The listing builds one solid part. Answer for the finished solid, in the listing's coordinates (mm). Face numbers are marked on the shaded views. Round coordinates to 2 decimals unless told otherwise and drop trailing zeros. Loops run counter-clockwise (first coordinate to the right, second up) from the corner with the lowest first, then second, coordinate; pieces in that order, holes last. Notation, with made-up numbers: M -21.75,-38 L 19.25,-38 A24 cw 19.25,-23 Z; hole C 25.5,11 d11. An arc over 180 degrees is marked long. Put each result on its own line as item: value. Start each with the question number.
(1) Straight lines are drawn through the part: line 1 (X direction, y = 5, z = 18); line 2 (X direction, y = 13.25, z = -47); line 3 (X direction, y = 18.75, z = -24.5). For each, find the intervals that lie inside material, in ascending order.
(2) Determine the mould class of the marked faces 1 and 2 for opening direction X: released by +X, released by -X, zero draft, split by the parting line, or undercut.
(3) Section B-B, the plane x = 0 is taken. Determine the outline of the cut face in (y, z).
(4) Flat-ended cylindrical pins translate along their axes: P1, Ø1, axis at x = 36.5, y = 6.5, coming from the +Z side; P2, Ø1, axis at x = -95.5, z = -94.5, coming from the +Y side; P3, Ø5, axis at y = 13.5, z = 75, coming from the +X side. Find the tip coordinate at first contact, or state that the pin passes through.
(5) Section A-A, the plane y = 18.25 is taken. Determine the outline of the cut face in (x, z).
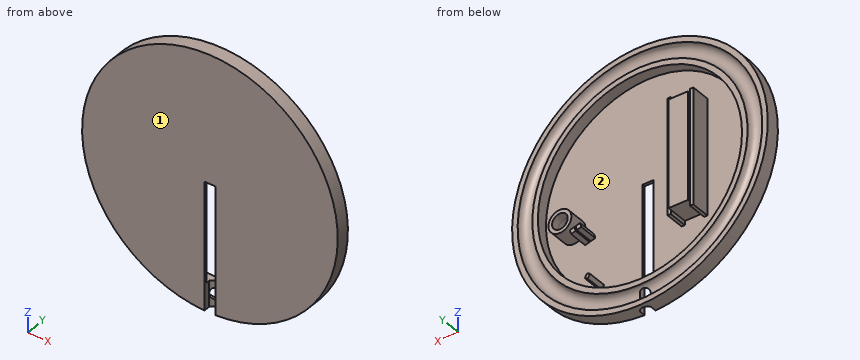
```python
from build123d import *

# Parameters (mm, degrees)
SKETCH1_W                = 139
SKETCH1_H                = 15
SKETCH4_W                = 21
SKETCH4_H                = 117
BOSS_EXTRUDE1_DEPTH      = 12
SKETCH5_R                = 12.5
SKETCH5_R_2              = 8.5
BOSS_EXTRUDE2_DEPTH      = 8.8
BOSS_EXTRUDE3_DEPTH      = 8.8
SKETCH11_W               = 28
SKETCH11_H               = 126
SKETCH11_W_2             = 21
SKETCH11_H_2             = 117
BOSS_EXTRUDE5_DEPTH      = 8.8
CUT_EXTRUDE1_START       = -12
SKETCH13_R               = 111
SKETCH13_R_2             = 12.5
SKETCH13_W               = 28
SKETCH13_H               = 126
SKETCH13_R_3             = 8.5
CUT_EXTRUDE1_DEPTH       = 12
BOSS_EXTRUDE6_DEPTH      = 8.8
BOSS_EXTRUDE6_DEPTH_BACK = 12
SKETCH14_W               = 21
SKETCH14_H               = 4.5
CUT_EXTRUDE2_DEPTH       = 20.8
CUT_EXTRUDE3_START       = -139
CUT_EXTRUDE3_DEPTH       = 139


# Read off the part's stored shape, not the designer's step: Cut-Extrude3
with BuildPart() as part:
    # Sketch1 → Revolve1 (revolve)
    with BuildSketch(Plane.XY, mode=Mode.PRIVATE) as revolve1_sk:
        with Locations((69.5, 7.5)):
            Rectangle(SKETCH1_W, SKETCH1_H)
    revolve(revolve1_sk.sketch.rotate(Axis((0, 4.511025306, 0), (0, 1, 0)), 90), axis=Axis((0, 4.511025306, 0), (0, 1, 0)))

    # Sketch4 → Boss-Extrude1 (add)
    with BuildSketch(Plane(origin=(0, 15, 0), x_dir=(1, 0, 0), z_dir=(0, 1, 0))):
        with Locations((-50.5, 0)):
            Rectangle(SKETCH4_W, SKETCH4_H)
    extrude(amount=BOSS_EXTRUDE1_DEPTH)

    # Sketch5 → Boss-Extrude2 (add)
    with BuildSketch(Plane(origin=(0, 15, 0), x_dir=(1, 0, 0), z_dir=(0, 1, 0))):
        with Locations(Location((80.590940898, 19.851958221, 0), (0, 0, 270))):
            Circle(SKETCH5_R)
        with Locations(Location((80.590940898, 19.851958221, 0), (0, 0, 270))):
            Circle(SKETCH5_R_2, mode=Mode.SUBTRACT)
    extrude(amount=BOSS_EXTRUDE2_DEPTH)

    # Sketch9 → Boss-Extrude3 (add)
    with BuildSketch(Plane(origin=(0, 15, 0), x_dir=(1, 0, 0), z_dir=(0, 1, 0))):
        with BuildLine():
            Line((47.886099404, 90.060654472), (50.233457218, 94.475392436))
            ThreePointArc((50.233457218, 94.475392436), (51.874629366, 93.584308664), (53.5, 92.664718205))
            Line((53.5, 92.664718205), (51, 88.334591186))
            ThreePointArc((51, 88.334591186), (49.450581265, 89.211210128), (47.886099404, 90.060654472))
        make_face()
    extrude(amount=BOSS_EXTRUDE3_DEPTH)

    # Sketch11 → Boss-Extrude5 (add)
    with BuildSketch(Plane(origin=(0, 15, 0), x_dir=(1, 0, 0), z_dir=(0, 1, 0))):
        with Locations((-50.5, 0)):
            Rectangle(SKETCH11_W, SKETCH11_H)
        with Locations((-50.5, 0)):
            Rectangle(SKETCH11_W_2, SKETCH11_H_2, mode=Mode.SUBTRACT)
    extrude(amount=BOSS_EXTRUDE5_DEPTH)

    # Sketch13 → Cut-Extrude1 (cut)
    # profile 1 of 2: a face of its own
    with BuildSketch(Plane(origin=(0, 15, 0), x_dir=(1, 0, 0), z_dir=(0, 1, 0)).offset(CUT_EXTRUDE1_START)):
        with Locations(Location((0, 0, 0), (0, 0, 270))):
            Circle(SKETCH13_R)
        with Locations(Location((80.590940898, 19.851958221, 0), (0, 0, 90))):
            Circle(SKETCH13_R_2, mode=Mode.SUBTRACT)
        with BuildLine():
            ThreePointArc((50.233457218, 94.475392436), (51.874629366, 93.584308664), (53.5, 92.664718205))
            Line((53.5, 92.664718205), (51, 88.334591186))
            ThreePointArc((51, 88.334591186), (49.450581265, 89.211210128), (47.886099404, 90.060654472))
            Line((47.886099404, 90.060654472), (50.233457218, 94.475392436))
        make_face(mode=Mode.SUBTRACT)
        with Locations((-50.5, 0)):
            Rectangle(SKETCH13_W, SKETCH13_H, mode=Mode.SUBTRACT)
    # profile 2 of 2: a face of its own
    with BuildSketch(Plane(origin=(0, 15, 0), x_dir=(1, 0, 0), z_dir=(0, 1, 0)).offset(CUT_EXTRUDE1_START)):
        with Locations(Location((80.590940898, 19.851958221, 0), (0, 0, 90))):
            Circle(SKETCH13_R_3)
    extrude(amount=CUT_EXTRUDE1_DEPTH, mode=Mode.SUBTRACT)

    # Sketch12 → Boss-Extrude6 (add, two sides: drawn at the far end of the back side and taken through both)
    with BuildSketch(Plane(origin=(0, 15, 0), x_dir=(1, 0, 0), z_dir=(0, 1, 0)).offset(-BOSS_EXTRUDE6_DEPTH_BACK)):
        Polygon((64.928294207, 32.551017187), (63.606991435, 37.373273815), (68.429248063, 38.694576587), (69.750550835, 33.872319959), align=None)
        Polygon((63.481617219, 32.154626355), (62.160314446, 36.976882983), (57.338057819, 35.655580211), (58.659360591, 30.833323583), align=None)
    extrude(amount=BOSS_EXTRUDE6_DEPTH + BOSS_EXTRUDE6_DEPTH_BACK)

    # Sketch14 → Cut-Extrude2 (cut)
    with BuildSketch(Plane(origin=(0, 23.8, 0), x_dir=(1, 0, 0), z_dir=(0, 1, 0))):
        with Locations((-50.5, -60.75)):
            Rectangle(SKETCH14_W, SKETCH14_H)
        with Locations((-50.5, 60.75)):
            Rectangle(SKETCH14_W, SKETCH14_H)
    extrude(amount=-CUT_EXTRUDE2_DEPTH, mode=Mode.SUBTRACT)

    # Cut-Extrude3 outline → Cut-Extrude3 (cut)
    with BuildSketch(Plane.XY.offset(CUT_EXTRUDE3_START)):
        with BuildLine():
            ThreePointArc((5.848066516, 0), (5.925428493, 0.127755535), (6, 0.257159717))
            Line((6, 0.257159717), (6, 7))
            ThreePointArc((6, 7), (0, 10.510910407), (-6, 7))
            Line((-6, 7), (-6, 0.257159717))
            ThreePointArc((-6, 0.257159717), (-5.925428493, 0.127755535), (-5.848066516, 0))
            Line((-5.848066516, 0), (5.848066516, 0))
        make_face()
    extrude(amount=CUT_EXTRUDE3_DEPTH, mode=Mode.SUBTRACT)

    # Sketch2 → Cut-Revolve1 (revolve, cut)
    with BuildSketch(Plane.XY, mode=Mode.PRIVATE) as cut_revolve1_sk:
        with BuildLine():
            Line((117, 15), (133, 15))
            ThreePointArc((133, 15), (125, 7), (117, 15))
        make_face()
    revolve(cut_revolve1_sk.sketch.rotate(Axis((0, 15, 0), (0, 1, 0)), 270), axis=Axis((0, 15, 0), (0, 1, 0)), mode=Mode.SUBTRACT)


solid = part.part
```
Recorded:
1. line 1: x = -137.83 to -109.53, -64.5 to -36.5, 109.53 to 137.83
1. line 2: x = -130.81 to -124.21, -107.36 to -100.56, -64.5 to -36.5, 100.56 to 107.36, 124.21 to 130.81
1. line 3: x = -64.5 to -36.5, 68.99 to 73.47, 87.71 to 92.19
2. face 1: zero draft
2. face 2: undercut
3. outline: M 0,0 L 3,0 L 3,111 L 15,111 L 15,117 A8 cw 15,133 L 15,139 L 0,139 Z; M 10.51,-139 L 15,-139 L 15,-133 A8 cw 10.51,-131.62 Z; M 10.51,-118.38 A8 cw 15,-117 L 15,-111 L 10.51,-111 Z
4. P1: stops at z = 134.26
4. P2: stops at y = 15
4. P3: stops at x = 118.59
5. outline: M -64.5,-63 L -61,-63 L -61,-58.5 L -40,-58.5 L -40,-63 L -36.5,-63 L -36.5,63 L -40,63 L -40,58.5 L -61,58.5 L -61,63 L -64.5,63 Z; M 47.89,-90.06 L 50.23,-94.48 A107 ccw 53.5,-92.66 L 51,-88.33 A102 cw Z; M 57.34,-35.66 L 62.16,-36.98 L 63.48,-32.15 L 58.66,-30.83 Z; M 63.61,-37.37 L 68.43,-38.69 L 69.75,-33.87 L 64.93,-32.55 Z; C 80.59,-19.85 d25; hole C 80.59,-19.85 d17
